```python
from build123d import *

# Parameters (mm, degrees)
ESQUISSE2_W                  = 3.3
ESQUISSE2_H                  = 16.393670871
R_P_TITION_CIRCULAIRE1_COUNT = 2
R_P_TITION_CIRCULAIRE1_ANGLE = 120


with BuildPart() as part:
    # Esquisse1 → Révolution1 (revolve)
    with BuildSketch(Plane(origin=(0, 0, 0), x_dir=(0, 0, -1), z_dir=(1, 0, 0)), mode=Mode.PRIVATE) as r_volution1_sk:
        with BuildLine():
            Line((2.449489743, 12), (10.4, 12))
            ThreePointArc((10.4, 12), (10.824264069, 11.824264069), (11, 11.4))
            Line((11, 11.4), (11, 8.1))
            ThreePointArc((11, 8.1), (10.824264069, 7.675735931), (10.4, 7.5))
            Line((10.4, 7.5), (-15.4, 7.5))
            ThreePointArc((-15.4, 7.5), (-15.824264069, 7.675735931), (-16, 8.1))
            Line((-16, 8.1), (-16, 11.4))
            ThreePointArc((-16, 11.4), (-15.824264069, 11.824264069), (-15.4, 12))
            Line((-15.4, 12), (-2.449489743, 12))
            ThreePointArc((-2.449489743, 12), (0, 11), (2.449489743, 12))
        make_face()
    revolve(r_volution1_sk.sketch.rotate(Axis((0, 0, 2.449489743), (0, 0, -1)), 90), axis=Axis((0, 0, 2.449489743), (0, 0, -1)))

    # Esquisse2 → Dégagement M61 (revolve, cut)
    with BuildSketch(Plane(origin=(0, 0, 10), x_dir=(0, 0, -1), z_dir=(1, 0, 0))):
        with Locations((1.65, 8.196835436)):
            Rectangle(ESQUISSE2_W, ESQUISSE2_H)
    d_gagement_m61 = revolve(axis=Axis((0, -6.35, 10), (0, 1, 0)), mode=Mode.SUBTRACT)

    # Répétition circulaire1: Dégagement M61 ×2 about axis
    r_p_tition_circulaire1_axis = Axis((0, 0, 2.449489743), (0, 0, -1))
    for i in range(1, R_P_TITION_CIRCULAIRE1_COUNT):
        add(d_gagement_m61.rotate(r_p_tition_circulaire1_axis, i * R_P_TITION_CIRCULAIRE1_ANGLE / (R_P_TITION_CIRCULAIRE1_COUNT - 1)), mode=Mode.SUBTRACT)


solid = part.part
```
Read the model definition and answer for the solid it produces. Units are mm, in the model's axes. Round coordinates to 2 decimals unless told otherwise and drop trailing zeros. Write each loop counter-clockwise with the first axis right and the second up, starting at its lowest first coordinate (ties: lowest second). Pieces come first, ordered by that corner, then holes. Notation, with made-up numbers: (44, -16) -> (72, -16) arc R22 cw to (72, 5) -> close; hole circle Ø10 at (53, 60.5). An arc over 180 degrees is marked (long way). Answer in a Markdown table with one row per item. Add a question column.
1) Determine the mould class of faces 1 (the face through (3, -8, 16)), 2 (the face through (11.446, -3.604, -6.48)), 3 (the face through (-0.1, 9.4, 13.3)), 4 (the face through (-3, -8, -11)) for opening direction Z: pulls with the +Z half, pulls with the -Z half, needs draft (parallel to the pull), parting line crosses it, or undercut.
2) Find section D-D, the plane z = 5. Determine the outline of the cut face in (x, y), and give its area (3 significant figures).
3) Consider line 1 (Y direction, x = 0, z = 4); line 2 (Z direction, x = 0, y = 8.55); line 3 (Y direction, x = -4.5, z = 2.5). Determine where each line is inside the solid, lowest interval first.
4) Find section B-B, the plane y = 0. Determine the outline of the cut face in (x, z), and give its area (3 significant figures).
5) Find section C-C, the plane z = 10. Determine the outline of the cut face in (x, y).
6) Given P1, Ø12, axis at y = 9.5, z = 12, coming from the +X side; P2, Ø3, axis at y = -6, z = 3.5, coming from the -X side; P3, Ø4, axis at x = 9.5, z = 9.5, coming from the -Y side; P4, Ø8, axis at x = -2, z = -5, coming from the +Y side, each flat-ended and moving along its own axis, determine where each tip first touches the part or whether it passes through.
7) Find section A-A, the plane x = 0. Determine the outline of the cut face in (y, z).
Findings below:
| question | item | result |
|---|---|---|
| 1 | face 1 | pulls with the +Z half |
| 1 | face 2 | needs draft |
| 1 | face 3 | undercut |
| 1 | face 4 | pulls with the -Z half |
| 2 | outline | circle Ø24 at (0, 0); hole circle Ø15 at (0, 0) |
| 2 | area | 276 mm² |
| 3 | line 1 | -12 to -7.5, 7.5 to 12 |
| 3 | line 2 | -11 to 6.7, 13.3 to 16 |
| 3 | line 3 | -11.12 to -6, 6 to 11.12 |
| 4 | outline | (-12, -10.4) arc R0.6 ccw to (-11.4, -11) -> (-8.1, -11) arc R0.6 ccw to (-7.5, -10.4) -> (-7.5, 15.4) arc R0.6 ccw to (-8.1, 16) -> (-11.4, 16) arc R0.6 ccw to (-12, 15.4) -> (-12, 2.45) arc R3.5 cw to (-12, -2.45) -> close; (7.5, -10.4) arc R0.6 ccw to (8.1, -11) -> (11.4, -11) arc R0.6 ccw to (12, -10.4) -> (12, -2.45) arc R3.5 cw to (12, 2.45) -> (12, 15.4) arc R0.6 ccw to (11.4, 16) -> (8.1, 16) arc R0.6 ccw to (7.5, 15.4) -> close |
| 4 | area | 236 mm² |
| 5 | outline | (-3.3, 6.73) -> (-3.3, 11.54) arc R12 ccw (long way) to (8.34, -8.63) -> (4.18, -6.23) arc R7.5 cw (long way) to start; (3.3, 6.73) arc R7.5 cw to (7.48, -0.51) -> (11.64, -2.91) arc R12 ccw to (3.3, 11.54) -> close |
| 6 | P1 | x = 11.48 |
| 6 | P2 | x = -11.12 |
| 6 | P3 | y = -9.37 |
| 6 | P4 | y = 12 |
| 7 | outline | (-12, -10.4) arc R0.6 ccw to (-11.4, -11) -> (-8.1, -11) arc R0.6 ccw to (-7.5, -10.4) -> (-7.5, 15.4) arc R0.6 ccw to (-8.1, 16) -> (-11.4, 16) arc R0.6 ccw to (-12, 15.4) -> (-12, 2.45) arc R3.5 cw to (-12, -2.45) -> close; (7.5, -10.4) arc R0.6 ccw to (8.1, -11) -> (11.4, -11) arc R0.6 ccw to (12, -10.4) -> (12, -2.45) arc R3.5 cw to (12, 2.45) -> (12, 6.7) -> (7.5, 6.7) -> close; (7.5, 13.3) -> (12, 13.3) -> (12, 15.4) arc R0.6 ccw to (11.4, 16) -> (8.1, 16) arc R0.6 ccw to (7.5, 15.4) -> close |
